from build123d import *

# Parameters (mm, degrees)
CROQUIS1_R              = 22.5
SALIENTE_EXTRUIR1_DEPTH = 10
CROQUIS2_R              = 26
SALIENTE_EXTRUIR2_DEPTH = 30
SALIENTE_EXTRUIR4_START = -20
SALIENTE_EXTRUIR4_DEPTH = 20
CROQUIS5_R              = 2.5
CORTAR_EXTRUIR1_DEPTH   = 10


with BuildPart() as part:
    # Croquis1 → Saliente-Extruir1 (new body)
    with BuildSketch(Plane.XY):
        Circle(CROQUIS1_R)
    extrude(amount=-SALIENTE_EXTRUIR1_DEPTH)

    # Croquis2 → Saliente-Extruir2 (add)
    with BuildSketch(Plane.XY):
        Circle(CROQUIS2_R)
    extrude(amount=SALIENTE_EXTRUIR2_DEPTH)

    # Croquis3 → Saliente-Extruir4 (add)
    with BuildSketch(Plane.XY.offset(30).offset(SALIENTE_EXTRUIR4_START)):
        with BuildLine():
            Line((-24, -10), (-40, -30))
            Line((-40, -30), (-40, -60))
            Line((-40, -60), (40, -60))
            Line((40, -60), (40, -30))
            Line((40, -30), (24, -10))
            ThreePointArc((24, -10), (0, -26), (-24, -10))
        make_face()
    extrude(amount=SALIENTE_EXTRUIR4_DEPTH)

    # Croquis5 → Cortar-Extruir1 (cut)
    with BuildSketch(Plane.XZ.offset(60)):
        with Locations((-30, 20)):
            Circle(CROQUIS5_R)
        with Locations((30, 20)):
            Circle(CROQUIS5_R)
        with Locations((0, 20)):
            Circle(CROQUIS5_R)
    extrude(amount=-CORTAR_EXTRUIR1_DEPTH, mode=Mode.SUBTRACT)


solid = part.part
Read the model definition and answer for the solid it produces. Units are mm, in the model's axes. A direction names the side the tool comes from. Round coordinates to 2 decimals unless told otherwise and drop trailing zeros. Order: outer loops, then holes, each group sorted by start corner. A loop starts at its lowest first (then second) coordinate and runs counter-clockwise, first axis right, second up. Notation, with made-up numbers: (18, -32.75) - (43, -32.75) arc R27 ccw to (43, -15.75) - close; hole circle Ø7 at (40.25, -6). An arc over 180 degrees is marked (long way). Use one line per item in the form item = value. Start each with the question number.
(1) The part is cut by section D-D (x = 0). Give the vertices of the cut face in (y, z), then the cut area to 3 significant figures.
(2) Determine the mould class of faces 4 (the face through (32, -20, 20)), 5 (the face through (-32, -20, 20)), 6 (the face through (-30.33, -55.07, 22.48)) for opening direction X: +X half, -X half, draft (parallel to the pull), parting line (faces both ways), or undercut.
(3) The part is cut by section A-A (z = 20). Give the vertices of the cut face in (x, y).
(4) Flat-ended cylindrical pins translate along their axes: pin 1 Ø25 at (x, y) = (-5.5, -25) entering from -Z; pin 2 Ø6 at (y, z) = (7.5, 4.5) entering from +X; pin 3 Ø3 at (x, z) = (-20.5, 15.5) entering from +Y; pin 4 Ø2.5 at (x, z) = (-1, 20) entering from -Y. Find the tip coordinate at first contact, or state that the pin passes through.
(5) Find the intervals of material crossed by line 1 along Z through (x, y) = (0, -54); line 2 along Y through (x, z) = (10, 13); line 3 along Z through (x, y) = (-16.5, -30), in increasing order. Write a range as from..to.
(6) The part is cut by section C-C (y = 0). Give the vertices of the cut face in (x, z), then the cut area to 3 significant figures.
(7) For faces 1 (the face through (-1, -60, 24)), 2 (the face through (-11.7, 19.4, 0)), 3 (the face through (-30, -50, 20)), determine the directions among +Z, -Z, +X, -X, +Y, -Y from which every point of the face is accessible in a straight line to the end or side of a thin tool.
(8) The part is cut by section B-B (x = -30). Give the vertices of the cut face in (y, z), then the cut area to 3 significant figures.
Checked values:
q1.outline = (-60, 10) - (-26, 10) - (-26, 0) - (-22.5, 0) - (-22.5, -10) - (22.5, -10) - (22.5, 0) - (26, 0) - (26, 30) - (-60, 30) - (-60, 22.5) - (-50, 22.5) - (-50, 17.5) - (-60, 17.5) - close
q1.area = 2,640 mm^2
q2.face_4 = +X half
q2.face_5 = -X half
q2.face_6 = undercut
q3.outline = (-40, -60) - (-32.5, -60) - (-32.5, -50) - (-27.5, -50) - (-27.5, -60) - (-2.5, -60) - (-2.5, -50) - (2.5, -50) - (2.5, -60) - (27.5, -60) - (27.5, -50) - (32.5, -50) - (32.5, -60) - (40, -60) - (40, -30) - (24, -10) arc R26 ccw (long way) to (-24, -10) - (-40, -30) - close
q4.pin_1 = -10
q4.pin_2 = 25.61
q4.pin_3 = 17.75
q4.pin_4 = -50
q5.line_1 = 10..17.5, 22.5..30
q5.line_2 = -60..24
q5.line_3 = 10..30
q6.outline = (-26, 0) - (-22.5, 0) - (-22.5, -10) - (22.5, -10) - (22.5, 0) - (26, 0) - (26, 30) - (-26, 30) - close
q6.area = 2,010 mm^2
q7.face_1 = +Z, -Z, +X, -X, -Y
q7.face_2 = -Z
q7.face_3 = -Y
q8.outline = (-60, 10) - (-17.5, 10) - (-17.5, 30) - (-60, 30) - (-60, 22.5) - (-50, 22.5) - (-50, 17.5) - (-60, 17.5) - close
q8.area = 800 mm^2
